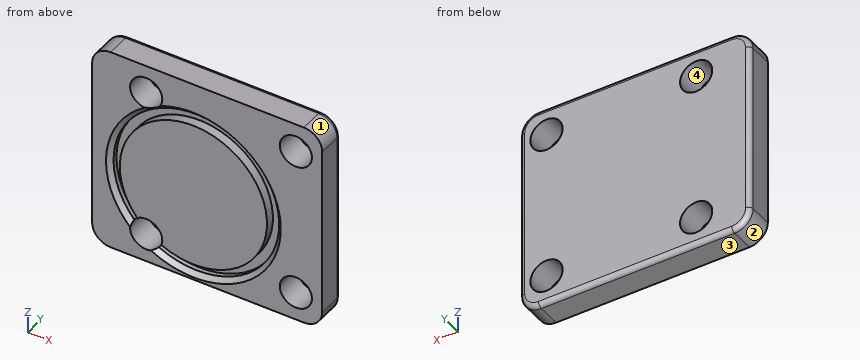
Autodesk Inventor part; units mm, degrees
ref_plane "YZ Plane" through (0, 0, 0) normal (1, 0, 0) x (0, 1, 0)
ref_plane "XZ Plane" through (0, 0, 0) normal (0, 1, 0) x (-1, 0, 0)
ref_plane "XY Plane" through (0, 0, 0) normal (0, 0, 1) x (1, 0, 0)
sketch "Sketch1" plane through (0, 0, 0) normal (0, 1, 0) x (-1, 0, 0)
  line L0 (25, -22.5) -> (-25, -22.5)
  line L1 (-25, -22.5) -> (-25, 22.5)
  line L2 (-25, 22.5) -> (25, 22.5)
  line L3 (25, 22.5) -> (25, -22.5)
  line L4 (25, -22.5) -> (-25, 22.5) construction
  line L5 (-25, -22.5) -> (25, 22.5) construction
  line L6 (0, 0) -> (-3, 0)
  circle A0 centre (-3, 0) radius 16
  line L7 (-3, 0) -> (-19.2635, -16.2635)
  line L8 (-3, 0) -> (20, 0) construction
  circle A1 centre (-19.2635, -16.2635) radius 3.5
  dimension "d0" = 50
  dimension "d1" = 45
  dimension "d35" = 0
  dimension "d36" = 3
  dimension "d37" = 32
  dimension "d38" = 23
  dimension "d39" = 135
  dimension "d40" = 7
extrude "Extrusion1" add sketch "Sketch1" along normal blind 6 contours L0 L1 L2 L3 | A0 | A1
fillet "Fillet1" radius 4 4 edges at (25, 3, 22.5) (25, 3, -22.5) (-25, 3, -22.5) (-25, 3, 22.5)
fillet "Fillet2" radius 1 8 edges at (23.8284, 6, 21.3284) (25, 6, 0) (23.8284, 6, -21.3284) (0, 6, -22.5) (-23.8284, 6, -21.3284) (-25, 6, 0) (-23.8284, 6, 21.3284) (0, 6, 22.5)
sketch "Sketch6" plane through (0, 0, 0) normal (0, -1, 0) x (1, 0, 0)
  circle A0 centre (-3, -3) radius 18
  point P0 (0, 0)
  dimension "d21" = 36
extrude "Extrusion6" cut sketch "Sketch6" against normal blind 2
sketch "Sketch7" plane through (-3, 2, -3) normal (0, -1, 0) x (1, 0, 0)
  circle A0 centre (0, 0) radius 16
  point P0 (3, 3)
  dimension "d27" = 32
extrude "Extrusion7" add sketch "Sketch7" along normal blind 2
chamfer "Chamfer1" distance 1 distance2 1 1 edges at (-21, 0, -3) measured on face at (21.6667, 0, -1)
sketch "Sketch10" plane through (0, 6, 0) normal (0, 1, 0) x (1, 0, 0)
  line L0 (0, 0) -> (3, 0)
  line L1 (3, 0) -> (19.2635, 16.2635)
  circle A0 centre (19.2635, 16.2635) radius 3.5
  dimension "d43" = 3
  dimension "d44" = 23
  dimension "d45" = 135
  dimension "d46" = 7
extrude "Extrusion8" cut sketch "Sketch10" against normal blind 10
sketch "Sketch11" plane through (0, 6, 0) normal (0, 1, 0) x (1, 0, 0)
  circle A0 centre (3, 0) radius 16
  point P0 (0, 0)
  dimension "d49" = 32
extrude "Extrusion9" cut sketch "Sketch11" against normal blind 2
pattern_circular "Circular Pattern2" count 4 over 360 about axis through (3, 6, 0) along (0, -1, 0) of "Extrusion8"
sketch "Sketch12" plane through (3, 4, 0) normal (0, 1, 0) x (1, 0, 0)
  circle A0 centre (0, 0) radius 16
  point P0 (-3, 0)
  dimension "d55" = 32
extrude "Extrusion10" add sketch "Sketch12" along normal blind 2
properties part number "cylinder head"
The model under review builds one solid part; all positions refer to its coordinate system, in mm. Face numbers are marked on the shaded views. Round coordinates to 2 decimals unless told otherwise and drop trailing zeros. Loops run counter-clockwise (first coordinate to the right, second up) from the corner with the lowest first, then second, coordinate; pieces in that order, holes last. Notation, with made-up numbers: M 87,64 L 144,64 A23 cw 144,92 Z; hole C 4,6 d10. An arc over 180 degrees is marked long. Answer as CSV lines item,"result". Start each with the question number.
Item 1: Consider section A-A (x = -3). Write out the cut boundary in (y, z), then the cut area to 3 significant figures.
Item 2: Insertion check: P1, Ø9, axis at x = -13.26, z = 16.26, coming from the -Y side. The pin has a flat end and moves straight along its axis. Give the tip position at first contact, or say it passes through.
Item 3: Consider section C-C (y = 2.75). Write out the cut boundary in (x, z), then the cut area to 3 significant figures.
Item 4: Mouldability with a two-part tool opening along X and no side actions: class the marked faces 1, 2, 3 and 4 as released by +X, released by -X, zero draft, split by the parting line, or undercut.
Item 5: Consider section B-B (z = -3). Write out the cut boundary in (x, y), then the cut area to 3 significant figures.
Item 6: Wall thickness on line 1 (X direction, y = 1.5, z = -3); line 2 (X direction, y = 5, z = 16.5); line 3 (Z direction, x = -3, y = 1.75): over which ranges is each line inside the solid? List them lowest first. Write a range as [from, to].
Answer:
1,outline,"M 0,-22.5 L 5,-22.5 A1 ccw 6,-21.5 L 6,21.5 A1 ccw 5,22.5 L 0,22.5 L 0,16 L 1,15 L 2,15 L 2,13 L 0,13 L 0,-19 L 2,-19 L 2,-21 L 1,-21 L 0,-22 Z"
1,area,"261 mm^2"
2,P1,"stops at y = 0"
3,outline,"M -25,-18.5 A4 ccw -21,-22.5 L 21,-22.5 A4 ccw 25,-18.5 L 25,18.5 A4 ccw 21,22.5 L -21,22.5 A4 ccw -25,18.5 Z; hole C -13.26,-16.26 d7; hole C -13.26,16.26 d7; hole C 19.26,-16.26 d7; hole C 19.26,16.26 d7"
3,area,"2,080 mm^2"
4,face 1,"released by +X"
4,face 2,"released by -X"
4,face 3,"zero draft"
4,face 4,"undercut"
5,outline,"M -25,0 L -22,0 L -21,1 L -21,2 L -19,2 L -19,0 L 13,0 L 13,2 L 15,2 L 15,1 L 16,0 L 25,0 L 25,5 A1 ccw 24,6 L -24,6 A1 ccw -25,5 Z"
5,area,"291 mm^2"
6,line 1,"x = [-25, -21], [-19, 13], [15, 25]"
6,line 2,"x = [-25, -16.76], [-9.77, 15.77], [22.76, 25]"
6,line 3,"z = [-22.5, -21], [-19, 13], [15, 22.5]"
